Could you check a few things on this model? Use its own coordinates, in mm. A direction names the side the tool comes from. Round coordinates to 2 decimals unless told otherwise and drop trailing zeros. Loops run counter-clockwise (first coordinate to the right, second up) from the corner with the lowest first, then second, coordinate; pieces in that order, holes last.
from build123d import *

# Parameters (mm, degrees)
F0_R     = 10
F0_W     = 8
F0_H     = 40
F0_R_2   = 30
F1_DEPTH = 8
F2_R     = 5


with BuildPart() as f1:
    # F0 (on Front) → F1 (new body)
    with BuildSketch(Plane.XZ):
        Polygon((-115.891304, -50), (-115.891304, -160), (204.108696, -160), (204.108696, -50), (73.341727, 0), (14.875664, 0), align=None)
        with Locations((-75.891304, -130)):
            Circle(F0_R, mode=Mode.SUBTRACT)
        with Locations((5.108696, -130)):
            Rectangle(F0_W, F0_H, mode=Mode.SUBTRACT)
        with Locations((83.108696, -130)):
            Rectangle(F0_W, F0_H, mode=Mode.SUBTRACT)
        with Locations((164.108696, -130)):
            Circle(F0_R, mode=Mode.SUBTRACT)
        with Locations((44.108696, -55)):
            Circle(F0_R_2, mode=Mode.SUBTRACT)
    extrude(amount=F1_DEPTH)

    # F2
    f2_edges = [f1.edges().sort_by_distance(p)[0] for p in [
        (-115.891304, -4, -50),
        (14.875664, -4, 0),
        (204.108696, -4, -50),
        (204.108696, -4, -160),
        (-115.891304, -4, -160),
        (73.341727, -4, 0),
    ]]
    fillet(f2_edges, radius=F2_R)


solid = f1.part
Item 1: If we section it at B-B, the plane y = -4.75: Please give me the cut outline in (x, z).
Results list:
outline: (-115.89, -155) arc R5 ccw to (-110.89, -160) - (199.11, -160) arc R5 ccw to (204.11, -155) - (204.11, -53.44) arc R5 ccw to (200.89, -48.77) - (74.2, -0.33) arc R5 ccw to (72.42, 0) - (15.8, 0) arc R5 ccw to (14.01, -0.33) - (-112.68, -48.77) arc R5 ccw to (-115.89, -53.44) - close; hole circle Ø20 at (-75.89, -130); hole (1.11, -150) - (9.11, -150) - (9.11, -110) - (1.11, -110) - close; hole circle Ø60 at (44.11, -55); hole (79.11, -150) - (87.11, -150) - (87.11, -110) - (79.11, -110) - close; hole circle Ø20 at (164.11, -130)
Item 2: If I drill on line 1 along X through (y, z) = (-3, -126); line 2 along X through (y, z) = (-6, -124.5); line 3 along Z through (x, y) = (41, -3.75), over which ranges is the centre line in solid material (lowest first)?
Results list:
line 1: x = -115.89 to -85.06, -66.73 to 1.11, 9.11 to 79.11, 87.11 to 154.94, 173.27 to 204.11
line 2: x = -115.89 to -84.24, -67.54 to 1.11, 9.11 to 79.11, 87.11 to 155.76, 172.46 to 204.11
line 3: z = -160 to -84.84, -25.16 to 0
Item 3: For faces 4 (the flat face through (5, -4, -150)), 5 (the flat face through (42, 0, -97)), which set-ups out of +Z, -Z, +X, -X, +Y, -Y let a thin tool reach every point of the face, with its end or its side?
Results list:
face 4: +Y, -Y
face 5: +Z, -Z, +X, -X, +Y
Item 4: If we section it at C-C, the plane x = 157.5: Please give me the cut outline in (y, z) (3 decimals), then the cut area to 3 significant figures.
Results list:
outline: (-8, -160) - (0, -160) - (0, -137.505) - (-8, -137.505) - close; (-8, -122.495) - (0, -122.495) - (0, -32.179) - (-8, -32.179) - close
area: 902 mm2
Item 5: If we section it at D-D, the plane z = -39.5: Please give me the cut outline in (x, y).
Results list:
outline: (-88.43, -8) - (18.42, -8) - (18.42, 0) - (-88.43, 0) - close; (69.79, -8) - (176.65, -8) - (176.65, 0) - (69.79, 0) - close
Item 6: We'd pull the mould along Z, two halves only. Please class faces 1 (the flat face through (42, -8, -97)), 2 (the flat face through (42, -4, -160)), 3 (the flat face through (9.109, -4, -130)): released by +Z, released by -Z, zero draft, split by the parting line, or undercut.
Results list:
face 1: zero draft
face 2: released by -Z
face 3: undercut
Item 7: If we section it at A-A, the plane z = -130: Please give me the cut outline in (x, y), then the cut area to 3 significant figures.
Results list:
outline: (-115.89, -8) - (-85.89, -8) - (-85.89, 0) - (-115.89, 0) - close; (-65.89, -8) - (1.11, -8) - (1.11, 0) - (-65.89, 0) - close; (9.11, -8) - (79.11, -8) - (79.11, 0) - (9.11, 0) - close; (87.11, -8) - (154.11, -8) - (154.11, 0) - (87.11, 0) - close; (174.11, -8) - (204.11, -8) - (204.11, 0) - (174.11, 0) - close
area: 2,110 mm2
Item 8: Will these pins go through, and if not, where does the flat tip stop? pin 1 (3 mm diameter, centred on x = 132, y = -1.5, fed in from +Z) (3 decimals); pin 2 (4 mm diameter, centred on x = 4.5, y = -5.5, fed in from +Z); pin 3 (16 mm diameter, centred on x = 164.11, z = -130, fed in from -Y); pin 4 (4 mm diameter, centred on x = 99.5, y = -4.5, fed in from +Z).
Results list:
pin 1: stops at z = -21.855
pin 2: stops at z = -3.2
pin 3: passes through
pin 4: stops at z = -9.24
